Build history of the part. All positions in model axes, mm. Round coordinates to 2 decimals unless told otherwise and drop trailing zeros. Loops run counter-clockwise (first coordinate to the right, second up) from the corner with the lowest first, then second, coordinate; pieces in that order, holes last. Notation, with made-up numbers: (65, 52.5) -> (108, 52.5) arc R28 ccw to (108, 78.5) -> close; hole circle Ø2 at (25, 71). An arc over 180 degrees is marked (long way). Put each result on its own line as item: value. Start each with the question number.
Item 1: Flat gauge pin, fed straight in: pin 1 Ø1 at (x, z) = (-2, 349.5) entering from +Y. Where does the tip first touch, or does it go through?
Item 2: Drill centre lines: probe 1 along Z at (x, y) = (0, -2.3); probe 2 along Y at (x, z) = (-4.5, 541); probe 3 along X at (y, z) = (-2.15, 7.5). Where is each one in solid material? Low to high. Write a range as [from, to].
Item 3: Cut at A-A, the plane y = 1. List the corners of the cut face in (x, z), plus the area to 3 significant figures.
Item 4: Cut at B-B, the plane z = 588. List the corners of the cut face in (x, y), plus the area to 4 significant figures.
```python
from build123d import *

# Parameters (mm, degrees)
EXTRUDE_1_DEPTH     = 655
CUT_EXTRUDE_1_REACH = 657.086
SKETCH_2_R          = 2.4


with BuildPart() as part:
    # ｽｹｯﾁ1 → ﾎﾞｽ - 押し出し1 (new body)
    with BuildSketch(Plane.XY):
        Polygon((-4.4, 3.1), (-4.4, 2.1), (-7.65, 2.1), (-7.65, -0.6), (7.65, -0.6), (7.65, 2.1), (4.4, 2.1), (4.4, 3.1), (8.65, 3.1), (8.65, -3.1), (-8.65, -3.1), (-8.65, 3.1), align=None)
    extrude(amount=EXTRUDE_1_DEPTH)

    # ｽｹｯﾁ2 → ｶｯﾄ - 押し出し1 (cut, up to next)
    with BuildSketch(Plane(origin=(0, -3.1, 0), x_dir=(-1, 0, 0), z_dir=(0, -1, 0)), mode=Mode.PRIVATE) as cut_extrude_1_sk1:
        with Locations(Location((0, -647.5, 0), (0, 0, 180))):
            Circle(SKETCH_2_R)
    cut_extrude_1_tool1 = extrude(cut_extrude_1_sk1.sketch, amount=-CUT_EXTRUDE_1_REACH, mode=Mode.PRIVATE) & part.part
    cut_extrude_1 = cut_extrude_1_tool1.solids().sort_by_distance((0, -3.1, 647.5))[0]
    add(cut_extrude_1, mode=Mode.SUBTRACT)

    # ﾐﾗｰ1: ｶｯﾄ - 押し出し1 across plane
    add(cut_extrude_1.mirror(Plane.XY.offset(327.5)), mode=Mode.SUBTRACT)


solid = part.part
```
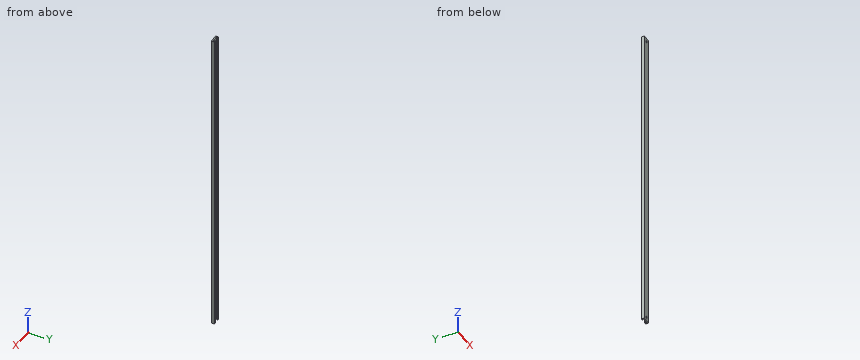
Reply:
1. pin 1: stops at y = -0.6
2. probe 1: z = [0, 5.1], [9.9, 645.1], [649.9, 655]
2. probe 2: y = [-3.1, -0.6], [2.1, 3.1]
2. probe 3: x = [-8.65, -2.4], [2.4, 8.65]
3. outline: (-8.65, 0) -> (-7.65, 0) -> (-7.65, 655) -> (-8.65, 655) -> close; (7.65, 0) -> (8.65, 0) -> (8.65, 655) -> (7.65, 655) -> close
3. area: 1,310 mm^2
4. outline: (-8.65, -3.1) -> (8.65, -3.1) -> (8.65, 3.1) -> (4.4, 3.1) -> (4.4, 2.1) -> (7.65, 2.1) -> (7.65, -0.6) -> (-7.65, -0.6) -> (-7.65, 2.1) -> (-4.4, 2.1) -> (-4.4, 3.1) -> (-8.65, 3.1) -> close
4. area: 57.15 mm^2
